from build123d import *

# Parameters (mm, degrees)
SKETCH1_W           = 16.5
SKETCH1_H           = 16.5
SKETCH1_R           = 1.15
BOSS_EXTRUDE1_DEPTH = 1.6
SKETCH2_W           = 3
SKETCH2_H           = 6.7
BOSS_EXTRUDE2_DEPTH = 2.3


with BuildPart() as part:
    # Sketch1 → Boss-Extrude1 (new body)
    with BuildSketch(Plane(origin=(0, 0, 0), x_dir=(1, 0, 0), z_dir=(0, 1, 0))):
        Rectangle(SKETCH1_W, SKETCH1_H)
        with Locations(Location((-5.75, 6, 0), (0, 0, 270))):
            Circle(SKETCH1_R, mode=Mode.SUBTRACT)
        with Locations(Location((5.75, 6, 0), (0, 0, 270))):
            Circle(SKETCH1_R, mode=Mode.SUBTRACT)
    extrude(amount=BOSS_EXTRUDE1_DEPTH)

    # Sketch2 → Boss-Extrude2 (add)
    with BuildSketch(Plane(origin=(0, 1.6, 0), x_dir=(1, 0, 0), z_dir=(0, 1, 0))):
        Rectangle(SKETCH2_W, SKETCH2_H)
    extrude(amount=BOSS_EXTRUDE2_DEPTH)


solid = part.part
Model file for the job. Use its own axes, mm. A direction names the side the tool comes from. Give positions to 0.01 mm unless a question says otherwise; leave off trailing zeros. Write each loop counter-clockwise with the first axis right and the second up, starting at its lowest first coordinate (ties: lowest second). Pieces come first, ordered by that corner, then holes. Notation, with made-up numbers: (80, 37.5) -> (110, 37.5) arc R21 cw to (110, 70.5) -> close; hole circle Ø1 at (81, 88). An arc over 180 degrees is marked (long way). Write item = value, one per line.
(1) Tool access for faces 1 (the face through (0, 3, 3.35)), 2 (the face through (0, 3, -3.35)), 3 (the face through (1.5, 3, 0)): list every direction of +Z, -Z, +X, -X, +Y, -Y with a clear straight run to the whole face (end or side of a thin tool).
Determined:
face_1 = +Z, +X, -X, +Y
face_2 = -Z, +X, -X, +Y
face_3 = +Z, -Z, +X, +Y
(2) Slice it at B-B, the plane z = -6. Give the cut face in (x, y), then the cut area to 3 significant figures.
Determined:
outline = (-8.25, 0) -> (-6.9, 0) -> (-6.9, 1.6) -> (-8.25, 1.6) -> close; (-4.6, 0) -> (4.6, 0) -> (4.6, 1.6) -> (-4.6, 1.6) -> close; (6.9, 0) -> (8.25, 0) -> (8.25, 1.6) -> (6.9, 1.6) -> close
area = 19.0 mm2
(3) Slice it at D-D, the plane y = 0.6. Give the cut face in (x, z).
Determined:
outline = (-8.25, -8.25) -> (8.25, -8.25) -> (8.25, 8.25) -> (-8.25, 8.25) -> close; hole circle Ø2.3 at (-5.75, -6); hole circle Ø2.3 at (5.75, -6)
(4) Probe line 1 along X through (y, z) = (0.8, -6); line 2 along Y through (x, z) = (5.25, -0.25); line 3 along Z through (x, y) = (-0.75, 1.9). List the from-to ranges inside material, lowest first.
Determined:
line_1 = -8.25 to -6.9, -4.6 to 4.6, 6.9 to 8.25
line_2 = 0 to 1.6
line_3 = -3.35 to 3.35
(5) Mould opens along Z. For faces 4 (the face through (6.527, 0.789, -6.848)), 5 (the face through (-1.5, 3, 0)), 6 (the face through (-4.973, 0.789, -6.848)), 7 (the face through (0, 1, -8.25)) say: released by +Z, released by -Z, zero draft, split by the parting line, or undercut.
Determined:
face_4 = undercut
face_5 = zero draft
face_6 = undercut
face_7 = released by -Z
(6) Slice it at A-A, the plane x = 5.75. Give the cut face in (y, z).
Determined:
outline = (0, -8.25) -> (1.6, -8.25) -> (1.6, -7.15) -> (0, -7.15) -> close; (0, -4.85) -> (1.6, -4.85) -> (1.6, 8.25) -> (0, 8.25) -> close
(7) Slice it at C-C, the plane z = 0.5. Give the cut face in (x, y).
Determined:
outline = (-8.25, 0) -> (8.25, 0) -> (8.25, 1.6) -> (1.5, 1.6) -> (1.5, 3.9) -> (-1.5, 3.9) -> (-1.5, 1.6) -> (-8.25, 1.6) -> close
(8) Flat gauge pins, fed straight in: P1, Ø1, axis at x = 1, y = 3, coming from the +Z side; P2, Ø0.7, axis at y = 2.5, z = 1.5, coming from the -X side. Where does each tip first touch, or does it go through?
Determined:
P1 = 3.35
P2 = -1.5
